```python
from build123d import *

# Parameters (mm, degrees)
F0_W     = 31.6
F0_H     = 57.7
F0_R     = 2
F1_DEPTH = 2
F2_R     = 1.5
F3_R     = 2


# Not quite as in the source:
# - a feature names something its author has since deleted; it is built from what else it names


with BuildPart() as f1:
    # F0 (on Top) → F1 (new body)
    with BuildSketch(Plane.XY):
        Rectangle(F0_W, F0_H)
        Polygon((7.8, 23.85), (13.8, 23.85), (13.8, 17.85), (13.8, -23.85), (-13.8, -23.85), (-13.8, 17.85), (-13.8, 23.85), (-7.8, 23.85), align=None, mode=Mode.SUBTRACT)
        Polygon((-15.8, -28.85), (-15.8, 28.85), (-25, -1), align=None)
        with Locations((-20, -1)):
            Circle(F0_R, mode=Mode.SUBTRACT)
        Polygon((25, -1), (15.8, 28.85), (15.8, -28.85), align=None)
        with Locations((20, -1)):
            Circle(F0_R, mode=Mode.SUBTRACT)
        Polygon((-13.8, 17.85), (-7.8, 23.85), (-13.8, 23.85), align=None)
        Polygon((13.8, 17.85), (13.8, 23.85), (7.8, 23.85), align=None)
    extrude(amount=F1_DEPTH)

    # F2
    f2_edges = [f1.edges().sort_by_distance(p)[0] for p in [
        (13.8, -23.85, 1),
        (-13.8, -23.85, 1),
    ]]
    fillet(f2_edges, radius=F2_R)

    # F3
    f3_edges = [f1.edges().sort_by_distance(p)[0] for p in [
        (15.8, -28.85, 1),
        (-15.8, -28.85, 1),
        (25, -1, 1),
        (15.8, 28.85, 1),
        (-15.8, 28.85, 1),
        (-25, -1, 1),
    ]]
    fillet(f3_edges, radius=F3_R)


solid = f1.part
```
Read the model definition and answer for the solid it produces. Units are mm, in the model's axes. A direction names the side the tool comes from. Coordinates: 2 decimals unless noted, no trailing zeros. Loops run counter-clockwise (first coordinate to the right, second up) from the corner with the lowest first, then second, coordinate; pieces in that order, holes last. Notation, with made-up numbers: (-32, 18.25) -> (-6, 18.25) arc R12 cw to (-6, 29.25) -> close; hole circle Ø5 at (22, 49). An arc over 180 degrees is marked (long way). Return JSON: item names as keys, results as strings.
Item 1: For faces 5 (the flat face through (0, 28.85, 1)), 6 (the flat face through (-13.8, -3, 1)), determine the directions among +Z, -Z, +X, -X, +Y, -Y from which every point of the face is accessible in a straight line to the end or side of a thin tool.
Answers:
{"face 5": "+Z, -Z, +X, -X, +Y", "face 6": "+Z, -Z"}
Item 2: Find section C-C (y = 10). Determine the outline of the cut face in (x, z).
Answers:
{"outline": "(-21.61, 0) -> (-13.8, 0) -> (-13.8, 2) -> (-21.61, 2) -> close; (13.8, 0) -> (21.61, 0) -> (21.61, 2) -> (13.8, 2) -> close"}
Item 3: For a pull along Y with two mould halves and no side action, classify faces 1 (the flat face through (-20.463, 13.719, 0.986)), 2 (the flat face through (0, -23.85, 1)), 3 (the flat face through (16, 0, 2)), 4 (the flat face through (-20.586, -14.361, 0.986)) as +Y half, -Y half, draft (parallel to the pull), parting line (faces both ways), or undercut.
Answers:
{"face 1": "+Y half", "face 2": "undercut", "face 3": "draft", "face 4": "-Y half"}
Item 4: Find the intervals of material crossed by probe 1 along Y at (x, z) = (1.5, 1.7); probe 2 along X at (y, z) = (-23, 1.45); probe 3 along X at (y, z) = (9, 1.95), in increasing order.
Answers:
{"probe 1": "y = -28.85 to -23.85, 23.85 to 28.85", "probe 2": "x = -17.73 to -13.65, 13.65 to 17.73", "probe 3": "x = -21.92 to -13.8, 13.8 to 21.92"}
Item 5: Find section A-A (z = 0.65). Determine the outline of the cut face in (x, y), plus the area to 3 significant figures.
Answers:
{"outline": "(-24.81, -0.39) arc R2 ccw to (-24.8, -1.61) -> (-16.25, -27.48) arc R2 ccw to (-14.35, -28.85) -> (14.35, -28.85) arc R2 ccw to (16.25, -27.48) -> (24.8, -1.61) arc R2 ccw to (24.81, -0.39) -> (16.23, 27.44) arc R2 ccw to (14.32, 28.85) -> (-14.32, 28.85) arc R2 ccw to (-16.23, 27.44) -> close; hole circle Ø4 at (-20, -1); hole (-13.8, -22.35) arc R1.5 ccw to (-12.3, -23.85) -> (12.3, -23.85) arc R1.5 ccw to (13.8, -22.35) -> (13.8, 17.85) -> (7.8, 23.85) -> (-7.8, 23.85) -> (-13.8, 17.85) -> close; hole circle Ø4 at (20, -1)", "area": "1,050 mm2"}
Item 6: Flat-ended cylindrical pins translate along their axes: P1, Ø5, axis at x = 20, y = -1, coming from the -Z side; P2, Ø0.6, axis at y = -0.5, z = 1.5, coming from the -X side; P3, Ø1, axis at y = 13.5, z = 1, coming from the -X side; P4, Ø1, axis at y = -11, z = 0.5, coming from the +X side. Find the tip coordinate at first contact, or state that the pin passes through.
Answers:
{"P1": "stops at z = 0", "P2": "stops at x = -24.89", "P3": "stops at x = -20.69", "P4": "stops at x = 21.86"}
Item 7: Find section B-B (x = 6). Determine the outline of the cut face in (y, z), plus the area to 3 significant figures.
Answers:
{"outline": "(-28.85, 0) -> (-23.85, 0) -> (-23.85, 2) -> (-28.85, 2) -> close; (23.85, 0) -> (28.85, 0) -> (28.85, 2) -> (23.85, 2) -> close", "area": "20.0 mm2"}
